from build123d import *

# Parameters (mm, degrees)
EXTRUDE_1_DEPTH             = 8
SKETCH_2_R                  = 2
EXTRUDE_2_DEPTH             = 6
SKETCH_3_R                  = 2
SKETCH_3_R_2                = 1.75
CUT_EXTRUDE_3_DEPTH         = 0.5
CHAMFER_1_SIZE              = 0.25
HOLE_WIZARD_M41_D           = 3.3
HOLE_WIZARD_M41_DEPTH       = 6
HOLE_WIZARD_M41_CSINK_D     = 4
HOLE_WIZARD_M41_CSINK_ANGLE = 90
HOLE_WIZARD_M41_TIP         = 0.991420021


with BuildPart() as part:
    # Эскиз1 → Вытянуть1 (new body)
    with BuildSketch(Plane.XY):
        Polygon((0, 4.041451884), (-3.5, 2.020725942), (-3.5, -2.020725942), (0, -4.041451884), (3.5, -2.020725942), (3.5, 2.020725942), align=None)
    extrude(amount=EXTRUDE_1_DEPTH)

    # Эскиз2 → Вытянуть2 (add)
    with BuildSketch(Plane.XY.offset(8)):
        Circle(SKETCH_2_R)
    extrude(amount=EXTRUDE_2_DEPTH)

    # Эскиз3 → Вырез-Вытянуть3 (cut)
    with BuildSketch(Plane.XY.offset(8)):
        Circle(SKETCH_3_R)
        Circle(SKETCH_3_R_2, mode=Mode.SUBTRACT)
    extrude(amount=CUT_EXTRUDE_3_DEPTH, mode=Mode.SUBTRACT)

    # Фаска1
    chamfer_1_edges = [part.edges().sort_by_distance(p)[0] for p in [
        (-2, 0, 14),
        (-2, 0, 8.5),
    ]]
    chamfer(chamfer_1_edges, length=CHAMFER_1_SIZE - 0.0001)  # a hair under: the kernel refuses the full size

    # Отверстие с зазором M41
    with Locations(Plane(origin=(0, 0, 0), x_dir=(-1, 0, 0), z_dir=(0, 0, -1))):
        with Locations((0, 0)):
            CounterSinkHole(HOLE_WIZARD_M41_D / 2, HOLE_WIZARD_M41_CSINK_D / 2, depth=HOLE_WIZARD_M41_DEPTH, counter_sink_angle=HOLE_WIZARD_M41_CSINK_ANGLE)
            with Locations((0, 0, -(HOLE_WIZARD_M41_DEPTH + HOLE_WIZARD_M41_TIP / 2))):  # 118° drill point
                Cone(0, HOLE_WIZARD_M41_D / 2, HOLE_WIZARD_M41_TIP, mode=Mode.SUBTRACT)


solid = part.part
Work out the finished part from the listing and answer in its coordinate system (mm). A direction names the side the tool comes from. Give positions to 0.01 mm unless a question says otherwise; leave off trailing zeros. Loops run counter-clockwise (first coordinate to the right, second up) from the corner with the lowest first, then second, coordinate; pieces in that order, holes last. Notation, with made-up numbers: (3, 12) -> (44, 12) arc R15 ccw to (44, 20) -> close; hole circle Ø2 at (-24, -32). An arc over 180 degrees is marked (long way). Use a Markdown table: item, result. Add a question column.
1. Flat-ended cylindrical pins translate along their axes: pin 1 Ø1.1 at (x, y) = (-0.5, 0) entering from -Z; pin 2 Ø4 at (y, z) = (1, 11) entering from +X; pin 3 Ø1.5 at (x, z) = (-1, 9) entering from +Y. Find the tip coordinate at first contact, or state that the pin passes through.
2. Determine the mould class of faces 1 (the conical face through (0.1, -0.3, 6.8)), 2 (the flat face through (1.726, -3.045, 3.944)), 3 (the flat face through (-2, -1, 8)) for opening direction X: released by +X, released by -X, zero draft, split by the parting line, or undercut.
3. Section C-C on x = 3.25 is taken. Determine the outline of the cut face in (y, z).
4. For faces 4 (the cylindrical face through (1.617, -0.67, 8.246)), 5 (the cylindrical face through (0, -2, 11)), 6 (the cylindrical face through (-1.216, 1.115, 3.215)), determine the directions among +Z, -Z, +X, -X, +Y, -Y from which every point of the face is accessible in a straight line to the end or side of a thin tool.
5. Find the intervals of material crossed by probe 1 along X at (y, z) = (0, 4.35); probe 2 along Z at (x, y) = (0.5, 3.5); probe 3 along Y at (x, z) = (1, 5.5), in increasing order.
6. Section A-A on z = 3.25 is taken. Determine the outline of the cut face in (x, y).
7. Section B-B on z = 10.5 is taken. Determine the outline of the cut face in (x, y).
Results below:
| question | item | result |
|---|---|---|
| 1 | pin 1 | stops at z = 6.36 |
| 1 | pin 2 | stops at x = 2 |
| 1 | pin 3 | stops at y = 1.98 |
| 2 | face 1 | undercut |
| 2 | face 2 | released by +X |
| 2 | face 3 | zero draft |
| 3 | outline | (-2.17, 0) -> (2.17, 0) -> (2.17, 8) -> (-2.17, 8) -> close |
| 4 | face 4 | none |
| 4 | face 5 | +Z |
| 4 | face 6 | -Z |
| 5 | probe 1 | x = -3.5 to -1.65, 1.65 to 3.5 |
| 5 | probe 2 | z = 0 to 8 |
| 5 | probe 3 | y = -3.46 to -1.31, 1.31 to 3.46 |
| 6 | outline | (-3.5, -2.02) -> (0, -4.04) -> (3.5, -2.02) -> (3.5, 2.02) -> (0, 4.04) -> (-3.5, 2.02) -> close; hole circle Ø3.3 at (0, 0) |
| 7 | outline | circle Ø4 at (0, 0) |
